Autodesk Fusion 360 part; units mm, degrees
sketch "Sketch1" plane through (0, 0, 0) normal (0, 0, 1) x (1, 0, 0)
  line L0 (0, -35) -> (0, -33.2289) construction
  line L1 (0, -33.2289) -> (0, 259.056) construction
  line L2 (-97.9811, 0) -> (484.4158, 0) construction
  line L3 (0, 0) -> (300, 0)
  line L4 (300, 0) -> (300, 200)
  line L5 (300, 200) -> (0, 200)
  line L6 (0, 200) -> (0, 0)
  line L7 (-60, 100) -> (400, 100) construction
  line L8 (25, 100) -> (25, 127.4792)
  line L9 (25, 100) -> (25, 72.5)
  line L10 (25, 127.4792) -> (80, 127.4792)
  line L11 (25, 72.5) -> (80, 72.5)
  line L12 (80, 127.4792) -> (80, 72.5)
  line L13 (21.5, 100) -> (21.5, 131) construction
  line L14 (21.5, 131) -> (83.5, 131) construction
  line L15 (21.4997, 69) -> (83.5, 69) construction
  circle A0 centre (52.5, 100) radius 31 construction
  circle A1 centre (52.5, 100) radius 27.5 construction
  line L16 (83.5, 131) -> (83.5, 69) construction
  line L17 (290, 69) -> (228, 69) construction
  line L18 (290, 100) -> (290, 69) construction
  line L19 (290, 100) -> (290, 131) construction
  line L20 (290, 131) -> (228, 131) construction
  line L21 (228, 131) -> (228, 69) construction
  line L22 (145, 126.7699) -> (90, 126.7699)
  line L23 (146, 151.2972) -> (93.5, 114.6946) construction
  line L24 (93.5, 114.6946) -> (93.5, 69) construction
  line L25 (146, 69) -> (93.5, 69) construction
  line L26 (146, 100) -> (146, 69) construction
  line L27 (146, 100) -> (146, 151.2972) construction
  line L28 (145, 71.7699) -> (90, 71.7699)
  line L29 (90, 126.7699) -> (90, 71.7699)
  line L30 (156, 131) -> (218, 131) construction
  line L31 (218, 131) -> (218, 69) construction
  line L32 (156, 100) -> (156, 131) construction
  line L33 (156, 100) -> (156, 69) construction
  line L34 (156, 69) -> (218, 69) construction
  line L35 (46, 37.5) -> (96, 37.5)
  line L36 (96, 7.5) -> (46, 7.5)
  line L37 (46, 7.5) -> (46, 37.5)
  line L38 (96, 37.5) -> (96, 7.5)
  line L39 (94, 6) -> (44, 6) construction
  line L40 (44, 6) -> (44, 39) construction
  line L41 (44, 39) -> (94, 39) construction
  line L42 (94, 39) -> (94, 6) construction
  line L43 (94, 6) -> (44, 39) construction
  line L44 (44, 6) -> (94, 39) construction
  line L45 (254, 37.5) -> (204, 37.5)
  line L46 (254, 7.5) -> (254, 37.5)
  line L47 (204, 7.5) -> (254, 7.5)
  line L48 (204, 37.5) -> (204, 7.5)
  circle A2 centre (38, 169) radius 2.75
  circle A3 centre (262, 169) radius 2.75
  line L49 (150, 200) -> (150, 0) construction
  line L50 (145, 126.7699) -> (145, 71.7699)
  line L51 (150, 190) -> (135, 190)
  line L52 (150, 190) -> (165, 190)
  line L53 (135, 190) -> (135, 160)
  line L54 (165, 190) -> (165, 160)
  line L55 (165, 160) -> (135, 160)
  line L56 (155, 126.7699) -> (155, 71.7699)
  line L57 (155, 126.7699) -> (210, 126.7699)
  line L58 (155, 71.7699) -> (210, 71.7699)
  line L59 (210, 126.7699) -> (210, 71.7699)
  line L60 (220, 127.4792) -> (220, 72.5)
  line L61 (275, 127.4792) -> (220, 127.4792)
  line L62 (275, 100) -> (275, 127.4792)
  line L63 (275, 100) -> (275, 72.5)
  line L64 (275, 72.5) -> (220, 72.5)
  line L65 (280, 200) -> (280, 0)
  line L66 (20, 200) -> (20, 0)
  point P0 (69, 22.5)
  dimension "d1" = 300
  dimension "d2" = 200
  dimension "d9" = 27.5
  dimension "d12" = 31
  dimension "d13" = 31
  dimension "d14" = 62
  dimension "d15" = 62
  dimension "d17" = 62
  dimension "d18" = 55
  dimension "d31" = 50
  dimension "d32" = 30
  dimension "d37" = 50
  dimension "d38" = 33
  dimension "d39" = 46
  dimension "d40" = 30
  dimension "d41" = 31.5
  dimension "d42" = 5.5
  dimension "d43" = 38
  dimension "d44" = 38
  dimension "d54" = 10
  dimension "d55" = 4
  dimension "d56" = 64
  dimension "d57" = 55
  dimension "d62" = 55
  dimension "d64" = 55
  dimension "d65" = 90
  dimension "d66" = 90
  dimension "d67" = 90
  dimension "d68" = 90
  dimension "d69" = 10
  dimension "d70" = 5
  dimension "d71" = 15
  dimension "d72" = 15
  dimension "d73" = 30
  dimension "d74" = 46
  dimension "d75" = 50
  dimension "d76" = 30
  dimension "d79" = 20
  dimension "d80" = 20
sketch "Sketch2" plane through (0, 0, 5) normal (0, 0, 1) x (-1, 0, 0)
  line L0 (-145, -71.7699) -> (-90, -71.7699)
  line L1 (-90, -71.7699) -> (-90, -126.7699)
  line L2 (-90, -126.7699) -> (-145, -126.7699)
  circle A0 centre (-38, -169) radius 2.75
  circle A1 centre (-262, -169) radius 2.75
  line L3 (-204, -7.5) -> (-204, -37.5)
  line L4 (-204, -37.5) -> (-254, -37.5)
  line L5 (-254, -37.5) -> (-254, -7.5)
  line L6 (-254, -7.5) -> (-204, -7.5)
  line L7 (-46, -37.5) -> (-96, -37.5)
  line L8 (-96, -37.5) -> (-96, -7.5)
  line L9 (-96, -7.5) -> (-46, -7.5)
  line L10 (-46, -7.5) -> (-46, -37.5)
  line L11 (-25, -72.5) -> (-25, -127.4792)
  line L12 (-25, -127.4792) -> (-80, -127.4792)
  line L13 (-80, -127.4792) -> (-80, -72.5)
  line L14 (-80, -72.5) -> (-25, -72.5)
  line L15 (0, -200) -> (0, 0)
  line L16 (0, 0) -> (-300, 0)
  line L17 (-300, 0) -> (-300, -200)
  line L18 (-300, -200) -> (0, -200)
  line L19 (0, -200) -> (0, 0)
  line L20 (-1, -200) -> (-1, 0)
  line L21 (-299, -200) -> (-299, 0)
  line L22 (-300, -200) -> (-300, 0)
  line L23 (-299, -200) -> (-300, -200)
  line L24 (-300, 0) -> (-299, 0)
  line L25 (-1, 0) -> (0, 0)
  line L26 (0, -200) -> (-1, -200)
  line L27 (-145, -126.7699) -> (-145, -71.7699)
  dimension "d49" = 1
  dimension "d50" = 1
sketch "Sketch5" plane through (0, 0, 0) normal (0, 0, 1) x (1, 0, 0)
  line L0 (20, 200) -> (20, 0)
  line L1 (0, -33.2289) -> (0, 259.056)
  line L2 (280, 200) -> (280, 0)
  line L3 (300, 0) -> (300, 200)
  dimension "d77" = 20
  dimension "d78" = 20
extrude "Extrude4" add sketch "Sketch1" along normal blind 4.5 contours L3 L5 L65 L66
sketch "Sketch6" plane through (0, 0, 4.5) normal (0, 0, 1) x (-1, 0, 0)
  circle A0 centre (-262, -169) radius 2.75
  line L0 (-90, -71.7699) -> (-90, -126.7699)
  line L1 (-90, -126.7699) -> (-145, -126.7699)
  line L2 (-145, -126.7699) -> (-145, -71.7699)
  line L3 (-145, -71.7699) -> (-90, -71.7699)
  line L4 (-25, -72.5) -> (-25, -127.4792)
  line L5 (-25, -127.4792) -> (-80, -127.4792)
  line L6 (-80, -127.4792) -> (-80, -72.5)
  line L7 (-80, -72.5) -> (-25, -72.5)
  line L8 (-46, -37.5) -> (-96, -37.5)
  line L9 (-96, -37.5) -> (-96, -7.5)
  line L10 (-96, -7.5) -> (-46, -7.5)
  line L11 (-46, -7.5) -> (-46, -37.5)
  line L12 (-204, -7.5) -> (-204, -37.5)
  line L13 (-204, -37.5) -> (-254, -37.5)
  line L14 (-254, -37.5) -> (-254, -7.5)
  line L15 (-254, -7.5) -> (-204, -7.5)
  line L16 (-135, -190) -> (-165, -190)
  line L17 (-165, -190) -> (-165, -160)
  line L18 (-165, -160) -> (-135, -160)
  line L19 (-135, -160) -> (-135, -190)
  circle A1 centre (-38, -169) radius 2.75
  line L20 (-155, -71.7699) -> (-155, -126.7699)
  line L21 (-155, -126.7699) -> (-210, -126.7699)
  line L22 (-210, -126.7699) -> (-210, -71.7699)
  line L23 (-210, -71.7699) -> (-155, -71.7699)
  line L24 (-275, -127.4792) -> (-275, -72.5)
  line L25 (-275, -72.5) -> (-220, -72.5)
  line L26 (-220, -72.5) -> (-220, -127.4792)
  line L27 (-220, -127.4792) -> (-275, -127.4792)
  line L28 (-280, -200) -> (-20, -200)
  line L29 (-20, -200) -> (-20, 0)
  line L30 (-20, 0) -> (-280, 0)
  line L31 (-280, 0) -> (-280, -200)
  line L32 (-23, -200) -> (-23, 0)
  line L33 (-277, -200) -> (-277, 0)
  line L34 (-23, -200) -> (-20, -200)
  line L35 (-20, -200) -> (-20, 0)
  line L36 (-23, 0) -> (-20, 0)
  line L37 (-277, 0) -> (-280, 0)
  line L38 (-280, 0) -> (-280, -200)
  line L39 (-277, -200) -> (-280, -200)
  dimension "d83" = 3
  dimension "d84" = 3
extrude "Extrude5" add sketch "Sketch6" against normal blind 95 contours L28 L30 L31 L33 L37 L38 L39 | L28 L29 L30 L32 L34 L35 L36
sketch "Sketch7" plane through (0, 0, 4.5) normal (0, 0, 1) x (-1, 0, 0)
  line L0 (-20, 0) -> (-280, 0)
  line L1 (-280, 0) -> (-280, -200)
  line L2 (-280, -200) -> (-20, -200)
  line L3 (-20, -200) -> (-20, 0)
  circle A0 centre (-262, -169) radius 2.75
  line L4 (-90, -71.7699) -> (-90, -126.7699)
  line L5 (-90, -126.7699) -> (-145, -126.7699)
  line L6 (-145, -126.7699) -> (-145, -71.7699)
  line L7 (-145, -71.7699) -> (-90, -71.7699)
  line L8 (-25, -72.5) -> (-25, -127.4792)
  line L9 (-25, -127.4792) -> (-80, -127.4792)
  line L10 (-80, -127.4792) -> (-80, -72.5)
  line L11 (-80, -72.5) -> (-25, -72.5)
  line L12 (-46, -37.5) -> (-96, -37.5)
  line L13 (-96, -37.5) -> (-96, -7.5)
  line L14 (-96, -7.5) -> (-46, -7.5)
  line L15 (-46, -7.5) -> (-46, -37.5)
  line L16 (-204, -7.5) -> (-204, -37.5)
  line L17 (-204, -37.5) -> (-254, -37.5)
  line L18 (-254, -37.5) -> (-254, -7.5)
  line L19 (-254, -7.5) -> (-204, -7.5)
  line L20 (-135, -190) -> (-165, -190)
  line L21 (-165, -190) -> (-165, -160)
  line L22 (-165, -160) -> (-135, -160)
  line L23 (-135, -160) -> (-135, -190)
  circle A1 centre (-38, -169) radius 2.75
  line L24 (-155, -71.7699) -> (-155, -126.7699)
  line L25 (-155, -126.7699) -> (-210, -126.7699)
  line L26 (-210, -126.7699) -> (-210, -71.7699)
  line L27 (-210, -71.7699) -> (-155, -71.7699)
  line L28 (-275, -127.4792) -> (-275, -72.5)
  line L29 (-275, -72.5) -> (-220, -72.5)
  line L30 (-220, -72.5) -> (-220, -127.4792)
  line L31 (-220, -127.4792) -> (-275, -127.4792)
  line L32 (-20, -4.5) -> (-280, -4.5)
  line L33 (-20, -195.5) -> (-280, -195.5)
  line L34 (-280, -195.5) -> (-280, -200)
  line L35 (-280, -200) -> (-20, -200)
  line L36 (-20, -195.5) -> (-20, -200)
  line L37 (-20, -4.5) -> (-20, 0)
  line L38 (-20, 0) -> (-280, 0)
  line L39 (-280, 0) -> (-280, -4.5)
  dimension "d87" = 4.5
  dimension "d88" = 4.5
extrude "Extrude6" add sketch "Sketch7" against normal blind 95 contours L0 L1 L3 L32 L37 L38 L39 | L1 L2 L3 L33 L34 L35 L36
sketch "Sketch8" plane through (0, 0, 0) normal (0, 0, -1) x (1, 0, 0)
  line L0 (275, -72.5) -> (275, -127.4792)
  line L1 (275, -127.4792) -> (220, -127.4792)
  line L2 (220, -127.4792) -> (220, -72.5)
  line L3 (220, -72.5) -> (275, -72.5)
  line L4 (155, -126.7699) -> (155, -71.7699)
  line L5 (155, -71.7699) -> (210, -71.7699)
  line L6 (210, -71.7699) -> (210, -126.7699)
  line L7 (210, -126.7699) -> (155, -126.7699)
  circle A0 centre (38, -169) radius 2.75
  line L8 (165, -190) -> (135, -190)
  line L9 (135, -190) -> (135, -160)
  line L10 (135, -160) -> (165, -160)
  line L11 (165, -160) -> (165, -190)
  line L12 (204, -37.5) -> (204, -7.5)
  line L13 (204, -7.5) -> (254, -7.5)
  line L14 (254, -7.5) -> (254, -37.5)
  line L15 (254, -37.5) -> (204, -37.5)
  line L16 (96, -37.5) -> (46, -37.5)
  line L17 (46, -37.5) -> (46, -7.5)
  line L18 (46, -7.5) -> (96, -7.5)
  line L19 (96, -7.5) -> (96, -37.5)
  line L20 (25, -127.4792) -> (25, -72.5)
  line L21 (25, -72.5) -> (80, -72.5)
  line L22 (80, -72.5) -> (80, -127.4792)
  line L23 (80, -127.4792) -> (25, -127.4792)
  line L24 (90, -126.7699) -> (90, -71.7699)
  line L25 (90, -71.7699) -> (145, -71.7699)
  line L26 (145, -71.7699) -> (145, -126.7699)
  line L27 (145, -126.7699) -> (90, -126.7699)
  circle A1 centre (262, -169) radius 2.75
  line L28 (277, -4.5) -> (23, -4.5)
  line L29 (23, -4.5) -> (23, -195.5)
  line L30 (23, -195.5) -> (277, -195.5)
  line L31 (277, -195.5) -> (277, -4.5)
  circle A2 centre (150, -100) radius 2
  circle A3 centre (150, -100) radius 0.5
  dimension "d91" = 1
extrude "Extrude7" add sketch "Sketch8" along normal blind 90 contours A2
sketch "Sketch9" plane through (0, 0, -90.5) normal (0, 0, -1) x (1, 0, 0)
  line L0 (277, -4.5) -> (277, -195.5)
  line L1 (277, -195.5) -> (23, -195.5)
  line L2 (23, -195.5) -> (23, -4.5)
  line L3 (23, -4.5) -> (277, -4.5)
  line L4 (280, 0) -> (20, 0)
  line L5 (20, 0) -> (20, -200)
  line L6 (20, -200) -> (280, -200)
  line L7 (280, -200) -> (280, 0)
  line L8 (271.3431, -4.5) -> (277, -10.1569)
  line L9 (23, -189.8431) -> (28.6569, -195.5)
  line L10 (23, -10.1569) -> (28.6569, -4.5)
  line L11 (277, -189.8431) -> (271.3431, -195.5)
  dimension "d94" = 45
  dimension "d96" = 45
  dimension "d98" = 45
  dimension "d99" = 45
  dimension "d100" = 45
  dimension "d101" = 8
  dimension "d102" = 8
  dimension "d104" = 8
  dimension "d105" = 8
extrude "Extrude8" add sketch "Sketch9" against normal blind 20 contours L0 L3 L8 | L0 L1 L11 | L2 L3 L10 | L1 L2 L9
Part model, mm, in its own coordinate system. A direction names the side the tool comes from. Round coordinates to 2 decimals unless told otherwise and drop trailing zeros. Write each loop counter-clockwise with the first axis right and the second up, starting at its lowest first coordinate (ties: lowest second). Pieces come first, ordered by that corner, then holes.
Item 1: Cut at C-C, the plane y = 18. Give the cut face in (x, z), plus the area to 3 significant figures.
Results:
outline: (20, -90.5) - (23, -90.5) - (23, 0) - (46, 0) - (46, 4.5) - (20, 4.5) - close; (96, 0) - (204, 0) - (204, 4.5) - (96, 4.5) - close; (254, 0) - (277, 0) - (277, -90.5) - (280, -90.5) - (280, 4.5) - (254, 4.5) - close
area: 1,260 mm2
Item 2: Two-plate mould, pull along Z, no slides. Class faces 1 (the flat face through (148, 101, 4.5)), 2 (the flat face through (25.789, 192.632, -80.64)), 3 (the flat face through (275, 194, -70.5)), 4 (the flat face through (151, 196, -90.5)): +Z half, -Z half, draft (parallel to the pull), parting line (faces both ways), or undercut.
Results:
face 1: +Z half
face 2: draft
face 3: undercut
face 4: -Z half
Item 3: Cut at D-D, the plane x = 196.5. Give the cut face in (y, z), plus the area to 3 significant figures.
Results:
outline: (0, -90.5) - (4.5, -90.5) - (4.5, 0) - (71.77, 0) - (71.77, 4.5) - (0, 4.5) - close; (126.77, 0) - (195.5, 0) - (195.5, -90.5) - (200, -90.5) - (200, 4.5) - (126.77, 4.5) - close
area: 1,470 mm2
Item 4: Which spindle directions (+Z, -Z, +X, -X, +Y, -Y) get a long thin tool onto all of the face, cutting with end or side? Do faces 5 (the flat face through (152, 200, -44)), 6 (the flat face through (275, 6, -70.5)), 7 (the flat face through (274.211, 192.632, -80.64)). Say none if no direction does.
Results:
face 5: +Z, -Z, +X, -X, +Y
face 6: none
face 7: -Z
Item 5: Cut at A-A, the plane z = -33.5. Give the cut face in (x, y).
Results:
outline: (20, 0) - (280, 0) - (280, 200) - (20, 200) - close; circle Ø4 at (150, 100); hole (23, 4.5) - (277, 4.5) - (277, 195.5) - (23, 195.5) - close; hole circle Ø1 at (150, 100)
Item 6: Cut at B-B, the plane x = 262. Give the cut face in (y, z), plus the area to 3 significant figures.
Results:
outline: (0, -90.5) - (4.5, -90.5) - (4.5, 0) - (72.5, 0) - (72.5, 4.5) - (0, 4.5) - close; (127.48, 0) - (166.25, 0) - (166.25, 4.5) - (127.48, 4.5) - close; (171.75, 0) - (195.5, 0) - (195.5, -90.5) - (200, -90.5) - (200, 4.5) - (171.75, 4.5) - close
area: 1,440 mm2
Item 7: Probe L1, parallel to X at y = 100, z = -51; L2, parallel to X at y = 169, z = 2; L3, parallel to Y at x = 38, z = 1. List the from-to ranges inside material, lowest first.
Results:
L1: x = 20 to 23, 148 to 149.5, 150.5 to 152, 277 to 280
L2: x = 20 to 35.25, 40.75 to 135, 165 to 259.25, 264.75 to 280
L3: y = 0 to 72.5, 127.48 to 166.25, 171.75 to 200
Item 8: Drop a flat-ended pin along its axis: pin 1 Ø4.5 at (x, y) = (38, 169) entering from +Z. Give the stop position or say it passes through.
Results:
pin 1: passes through
